Autodesk Inventor part; units mm, degrees
ref_plane "YZ Plane" through (0, 0, 0) normal (1, 0, 0) x (0, 1, 0)
ref_plane "XZ Plane" through (0, 0, 0) normal (0, 1, 0) x (-1, 0, 0)
ref_plane "XY Plane" through (0, 0, 0) normal (0, 0, 1) x (1, 0, 0)
sketch "Эскиз1" plane through (0, 0, 0) normal (0, 1, 0) x (-1, 0, 0)
  circle A0 centre (0, 0) radius 7.9
  circle A1 centre (0, 0) radius 2
  circle A2 centre (0, 0) radius 6
  dimension "d0" = 15.8
  dimension "d1" = 4
  dimension "d4" = 12
extrude "Выдавливание1" add sketch "Эскиз1" along normal mid plane 9.15 contours A0 | A2
extrude "Выдавливание2" cut sketch "Эскиз1" along normal mid plane 7.15 contours A0
properties part number "Pulley"
Check sheet for the modelled part. Datum: model origin and axes. Units: mm. A direction names the side the tool comes from. Coordinates: 2 decimals unless noted, no trailing zeros. Order: outer loops, then holes, each group sorted by start corner. A loop starts at its lowest first (then second) coordinate and runs counter-clockwise, first axis right, second up. Notation, with made-up numbers: M -11.5,48.5 L 0.5,48.5 A31 ccw 0.5,86.5 Z; hole C 71,-5 d1. An arc over 180 degrees is marked long. Write each question's results on one line, items separated by ' | '. Start each with the question number.
1. Cross-section at A-A on x = 0. Record the cut outline in (y, z) (3 decimals).
2. Material ranges on probe 1 along Y at (x, z) = (-6, -3) (3 decimals); probe 2 along Z at (x, y) = (0, -1.75); probe 3 along X at (y, z) = (1.75, 0.5), recorded low to high.
3. Go/stop test with flat-tipped pins: P1, Ø5, axis at x = 4, y = -1.5, coming from the -Z side; P2, Ø5, axis at y = 1.5, z = -3.5, coming from the +X side. Record where each tip stops, or that it passes through.
4. Mould release check, pull along Y, two halves, no side actions. Record for faces 1 (the face through (0, 0, 2)), 2 (the face through (-2, -4.575, -2)), 3 (the face through (6, 0, 0)): +Y half, -Y half, draft (parallel to the pull), parting line (faces both ways), or undercut.
5. Cross-section at C-C on y = 0.25. Record the cut outline in (x, z), and give its area (3 significant figures).
6. Cross-section at D-D on z = -5.25. Record the cut outline in (x, y) (3 decimals), and give its area (3 significant figures).
7. Cross-section at B-B on z = 0. Record the cut outline in (x, y) (3 decimals), and give its area (3 significant figures).
8. Access from +Z, -Z, +X, -X, +Y, -Y to the whole of each face (thin tool, end or side, straight path). Record for faces 4 (the face through (-2, 4.575, -2)), 5 (the face through (-2, -3.575, 6)).
Checks:
1) outline: M -4.575,-7.9 L -3.575,-7.9 L -3.575,-6 L 3.575,-6 L 3.575,-7.9 L 4.575,-7.9 L 4.575,-2 L -4.575,-2 Z; M -4.575,2 L 4.575,2 L 4.575,7.9 L 3.575,7.9 L 3.575,6 L -3.575,6 L -3.575,7.9 L -4.575,7.9 Z
2) probe 1: y = -4.575 to -3.575, 3.575 to 4.575 | probe 2: z = -6 to -2, 2 to 6 | probe 3: x = -5.98 to -1.94, 1.94 to 5.98
3) P1: stops at z = -7.46 | P2: stops at x = 7.61
4) face 1: draft | face 2: -Y half | face 3: undercut
5) outline: C 0,0 d12; hole C 0,0 d4 | area: 101 mm²
6) outline: M -5.903,-4.575 L 5.903,-4.575 L 5.903,-3.575 L 2.905,-3.575 L 2.905,3.575 L 5.903,3.575 L 5.903,4.575 L -5.903,4.575 L -5.903,3.575 L -2.905,3.575 L -2.905,-3.575 L -5.903,-3.575 Z | area: 65.2 mm²
7) outline: M -7.9,-4.575 L -2,-4.575 L -2,4.575 L -7.9,4.575 L -7.9,3.575 L -6,3.575 L -6,-3.575 L -7.9,-3.575 Z; M 2,-4.575 L 7.9,-4.575 L 7.9,-3.575 L 6,-3.575 L 6,3.575 L 7.9,3.575 L 7.9,4.575 L 2,4.575 Z | area: 80.8 mm²
8) face 4: +Z, -Z, +X, -X, +Y | face 5: none
